Geometry check sheet. Reference: the model listing, model coordinates, mm. A direction names the side the tool comes from. Give positions to 0.01 mm unless a question says otherwise; leave off trailing zeros. Loops run counter-clockwise (first coordinate to the right, second up) from the corner with the lowest first, then second, coordinate; pieces in that order, holes last. Notation, with made-up numbers: (-25, -8.5) -> (15, -8.5) arc R18 cw to (15, 7.5) -> close; hole circle Ø9 at (-34.75, 38.5). An arc over 180 degrees is marked (long way). Answer as a JSON object with one key per item and string values.
from build123d import *

# Parameters (mm, degrees)
F0_R      = 22.907165
F1_DEPTH  = 51.1
F4_DEPTH  = 106.8
F5_R      = 22.356235
F5_R_2    = 21
F6_DEPTH  = 54.8
F7_R      = 21.538885
F8_DEPTH  = 64.2
F9_W      = 6.154686
F9_H      = 33.235299
F9_W_2    = 5.339459
F9_H_2    = 37.849365
F10_DEPTH = 98.8
F11_DEPTH = 96.1


with BuildPart() as f1:
    # F0 (on Top) → F1 (new body)
    with BuildSketch(Plane.XY):
        Circle(F0_R)
    extrude(amount=F1_DEPTH)

    # F3 (on offset) → F4 (cut)
    with BuildSketch(Plane.YZ.offset(-32.2)):
        Polygon((-46.021562, 0), (31.365387, 56.67308), (-37.553031, 54.173857), align=None)
    extrude(amount=F4_DEPTH, mode=Mode.SUBTRACT)

    # F5 (on Top) → F6 (cut)
    with BuildSketch(Plane.XY):
        Circle(F5_R)
        Circle(F5_R_2, mode=Mode.SUBTRACT)
    extrude(amount=F6_DEPTH, mode=Mode.SUBTRACT)

    # F7 (on Top) → F8 (cut)
    with BuildSketch(Plane.XY):
        Circle(F7_R)
    extrude(amount=F8_DEPTH, mode=Mode.SUBTRACT)

    # F9 (on offset) → F10 (cut)
    with BuildSketch(Plane.YZ.offset(-32.2)):
        with Locations((-6.243853, 21.483376)):
            Rectangle(F9_W, F9_H)
        with Locations((6.204987, 23.790409)):
            Rectangle(F9_W_2, F9_H_2)
    extrude(amount=F10_DEPTH, mode=Mode.SUBTRACT)

    # F9 (on offset) → F11 (cut)
    with BuildSketch(Plane.YZ.offset(-32.2)):
        with Locations((-6.243853, 21.483376)):
            Rectangle(F9_W, F9_H)
        with Locations((6.204987, 23.790409)):
            Rectangle(F9_W_2, F9_H_2)
    extrude(amount=F11_DEPTH, mode=Mode.SUBTRACT)


solid = f1.part
1) Depth check by flat-ended pin: P1, Ø1.9, axis at x = -22, y = -6.5, coming from the +Z side; P2, Ø0.5, axis at x = 20.5, z = 17.5, coming from the +Y side; P3, Ø0.7, axis at x = 21, y = -6, coming from the +Z side; P4, Ø6, axis at y = 11.5, z = 8.5, coming from the +X side. Enter the tip coordinate at first touch or a pass-through.
Geometry check:
{"P1": "stops at z = 4.87", "P2": "stops at y = 10.71", "P3": "passes through", "P4": "stops at x = 21.12"}
2) Section check B-B on y = -8. Record the cut outline in (x, z).
Geometry check:
{"outline": "(-21.46, 0) -> (-20.88, 0) -> (-20.88, 4.87) -> (-21.46, 4.87) -> close; (20.88, 0) -> (21.46, 0) -> (21.46, 4.87) -> (20.88, 4.87) -> close"}
3) Section check D-D on z = 35. Record the cut outline in (x, y).
Geometry check:
{"outline": "(-22.84, 1.77) -> (-22.29, 1.77) arc R22.36 cw to (-22.07, 3.54) -> (-22.63, 3.54) arc R22.91 ccw to start; (-21.12, 8.87) -> (-20.52, 8.87) arc R22.36 cw to (20.52, 8.87) -> (21.12, 8.87) arc R22.91 ccw to start; (22.07, 3.54) arc R22.36 cw to (22.29, 1.77) -> (22.84, 1.77) arc R22.91 ccw to (22.63, 3.54) -> close"}
4) Draft check along X on faces 1 (the face through (5, -22, 0)), 2 (the face through (-16.477, 15.109, 19.123)), 3 (the face through (-16.884, 15.482, 19.277)). Enter one of: pulls with the +X half, pulls with the -X half, needs draft (parallel to the pull), parting line crosses it, or undercut.
Geometry check:
{"face 1": "needs draft", "face 2": "undercut", "face 3": "parting line crosses it"}
5) Section check C-C on x = -2. Record the cut outline in (y, z).
Geometry check:
{"outline": "(-22.82, 0) -> (-22.27, 0) -> (-22.27, 17.4) -> (-22.82, 16.99) -> close; (22.27, 0) -> (22.82, 0) -> (22.82, 50.41) -> (22.27, 50.01) -> close"}
6) Tool access check on faces 4 (the face through (22.578, 0.137, 33.804)), 5 (the face through (-21.7, 6.2, 4.866)). Record the directions out of +Z, -Z, +X, -X, +Y, -Y that give a thin tool (end or side, any length) a straight path to the whole face; none if there is none.
Geometry check:
{"face 4": "+Z, +X, -X, -Y", "face 5": "+Z, +X, -X"}
7) Material ranges on line 1 along Y through (x, z) = (0, 33); line 2 along Y through (x, z) = (3.5, 20); line 3 along X through (y, z) = (0, 21), recorded low to high. Write a range as from..to.
Geometry check:
{"line 1": "y = 22.36..22.91", "line 2": "y = 22.08..22.64", "line 3": "x = -22.91..-22.36, 22.36..22.91"}
8) Section check A-A on z = 12. Record the cut outline in (x, y).
Geometry check:
{"outline": "(-22.69, -3.17) -> (-22.13, -3.17) arc R22.36 cw to (-22.07, 3.54) -> (-22.63, 3.54) arc R22.91 ccw to start; (-21.12, 8.87) -> (-20.52, 8.87) arc R22.36 cw to (20.52, 8.87) -> (21.12, 8.87) arc R22.91 ccw to start; (-20.92, -9.32) arc R22.91 ccw to (20.92, -9.32) -> (20.32, -9.32) arc R22.36 cw to (-20.32, -9.32) -> close; (22.07, 3.54) arc R22.36 cw to (22.13, -3.17) -> (22.69, -3.17) arc R22.91 ccw to (22.63, 3.54) -> close"}
